Check sheet for the modelled part. Datum: model origin and axes. Units: mm. A direction names the side the tool comes from. Give positions to 0.01 mm unless a question says otherwise; leave off trailing zeros. Loops run counter-clockwise (first coordinate to the right, second up) from the corner with the lowest first, then second, coordinate; pieces in that order, holes last. Notation, with made-up numbers: (42, -4.5) -> (90, -4.5) arc R18 ccw to (90, 14.5) -> close; hole circle Ø9 at (47, 17). An arc over 180 degrees is marked (long way). Answer as CSV lines item,"result". Start each with the question number.
(1) Section check B-B on x = -46.5. Enter the section's corners in (y, z), plus the area to 3 significant figures.
(2) Access from +Z, -Z, +X, -X, +Y, -Y to the whole of each face (thin tool, end or side, straight path). Record for faces 4 (the face through (-45, -20, 40)), 5 (the face through (11, 7.5, 5)), 6 (the face through (10, 0, 45)).
(3) Gauge pin test, flat ends, axial feed: pin 1 Ø3 at (x, y) = (-44.5, 21) entering from -Z; pin 2 Ø8 at (y, z) = (-18.5, 42) entering from +X; pin 3 Ø10 at (x, y) = (40.5, -13) entering from +Z. Record the tip position at first contact, or that the pin passes through.
(4) Section check C-C on y = -17. Enter the section's corners in (x, z), plus the area to 3 significant figures.
(5) Release check for a two-part mould opening along Y. For faces 1 (the face through (-1, -25, 23)), 2 (the face through (9, -16, 0)), 3 (the face through (11, -7.5, 5)) record: pulls with the +Y half, pulls with the -Y half, needs draft (parallel to the pull), parting line crosses it, or undercut.
(6) Section check D-D on z = 50. Enter the section's corners in (x, y), plus the area to 3 significant figures.
(7) Material ranges on line 1 (X direction, y = -11, z = 57); line 2 (X direction, y = 9.5, z = 20.5); line 3 (Z direction, x = -9, y = 6.5), recorded low to high. Write a range as from..to.
(8) Section check A-A on z = 7. Enter the section's corners in (x, y), plus the area to 3 significant figures.
from build123d import *

# Parameters (mm, degrees)
F0_W     = 110
F0_H     = 50
F1_DEPTH = 60
F2_W     = 15
F2_H     = 20
F3_DEPTH = 110.001
F5_DEPTH = 30
F6_W     = 20
F6_H     = 40
F7_DEPTH = 50.001
F8_W     = 20
F8_H     = 30
F9_DEPTH = 60.001


with BuildPart() as f1:
    # F0 (on Top) → F1 (new body)
    with BuildSketch(Plane.XY):
        Rectangle(F0_W, F0_H)
    extrude(amount=F1_DEPTH)

    # F2 (on face) → F3 (cut, through all)
    with BuildSketch(Plane.YZ.offset(55)):
        Rectangle(F2_W, F2_H)
    extrude(amount=-F3_DEPTH, mode=Mode.SUBTRACT)

    # F4 (on face) → F5 (cut)
    with BuildSketch(Plane.XY.offset(60)):
        Polygon((55, 25), (25, 25), (25, 0), (-5, 0), (-5, -25), (55, -25), align=None)
    extrude(amount=-F5_DEPTH, mode=Mode.SUBTRACT)

    # F6 (on face) → F7 (cut, through all)
    with BuildSketch(Plane.XZ.offset(25)):
        with Locations((-45, 20)):
            Rectangle(F6_W, F6_H)
    extrude(amount=-F7_DEPTH, mode=Mode.SUBTRACT)

    # F8 (on face) → F9 (cut, through all)
    with BuildSketch(Plane.XY.offset(60)):
        with Locations((-45, 0)):
            Rectangle(F8_W, F8_H)
    extrude(amount=-F9_DEPTH, mode=Mode.SUBTRACT)


solid = f1.part
Working result:
1,outline,"(-25, 40) -> (-15, 40) -> (-15, 60) -> (-25, 60) -> close; (15, 40) -> (25, 40) -> (25, 60) -> (15, 60) -> close"
1,area,"400 mm^2"
2,face 4,"-Z, -X, +Y, -Y"
2,face 5,"-Z, +X, -X"
2,face 6,"+Z, +X, -Y"
3,pin 1,"stops at z = 40"
3,pin 2,"stops at x = -5"
3,pin 3,"stops at z = 30"
4,outline,"(-55, 40) -> (-35, 40) -> (-35, 0) -> (55, 0) -> (55, 30) -> (-5, 30) -> (-5, 60) -> (-55, 60) -> close"
4,area,"4,000 mm^2"
5,face 1,"pulls with the -Y half"
5,face 2,"needs draft"
5,face 3,"undercut"
6,outline,"(-55, -25) -> (-5, -25) -> (-5, 0) -> (25, 0) -> (25, 25) -> (-55, 25) -> (-55, 15) -> (-35, 15) -> (-35, -15) -> (-55, -15) -> close"
6,area,"2,650 mm^2"
7,line 1,"x = -35..-5"
7,line 2,"x = -35..55"
7,line 3,"z = 10..60"
8,outline,"(-35, -25) -> (55, -25) -> (55, -7.5) -> (-35, -7.5) -> close; (-35, 7.5) -> (55, 7.5) -> (55, 25) -> (-35, 25) -> close"
8,area,"3,150 mm^2"
